The listing builds one solid part. Answer for the finished solid, in the listing's coordinates (mm). A direction names the side the tool comes from. Coordinates: 2 decimals unless noted, no trailing zeros. Loops run counter-clockwise (first coordinate to the right, second up) from the corner with the lowest first, then second, coordinate; pieces in that order, holes last. Notation, with made-up numbers: (26.5, 46.5) - (63.5, 46.5) arc R16 cw to (63.5, 69.5) - close; hole circle Ø7 at (-30, 51.25). An arc over 180 degrees is marked (long way). Put each result on its own line as item: value.
```python
from build123d import *

# Parameters (mm, degrees)
SKETCH1_W                = 25.4
SKETCH1_H                = 76.2
BOSS_EXTRUDE1_DEPTH      = 25.4
SKETCH2_W                = 22.225
SKETCH2_H                = 22.225
CUT_EXTRUDE1_DEPTH       = 138.235224905
BOSS_EXTRUDE2_DEPTH      = 3.175
BOSS_EXTRUDE2_DEPTH_BACK = 31.75
SKETCH3_R                = 12.7
SKETCH4_R                = 3.175
CUT_EXTRUDE3_DEPTH       = 104.653950262


with BuildPart() as part:
    # Sketch1 → Boss-Extrude1 (new body)
    with BuildSketch(Plane(origin=(0, 0, 0), x_dir=(0, 0, -1), z_dir=(1, 0, 0))):
        Rectangle(SKETCH1_W, SKETCH1_H)
        Polygon((-12.7, -44.45), (-12.7, -38.1), (-12.7, 38.1), (-12.7, 63.5), (-14.2875, 63.5), (-14.2875, -44.45), align=None)
        Polygon((-12.7, -44.45), (-22.225, -94.650277885), (-23.784673135, -94.354345527), (-14.2875, -44.45), align=None)
        Polygon((22.225, -94.650277885), (23.784673135, -94.354345527), (14.2875, -44.45), (12.7, -44.45), align=None)
        Polygon((12.7, -38.1), (12.7, -44.45), (14.2875, -44.45), (14.2875, 63.5), (12.7, 63.5), (12.7, 38.1), align=None)
    extrude(amount=BOSS_EXTRUDE1_DEPTH)

    # Sketch2 → Cut-Extrude1 (cut, through all)
    with BuildSketch(Plane(origin=(0, 38.1, 0), x_dir=(1, 0, 0), z_dir=(0, 1, 0))):
        with Locations((12.7, 0)):
            Rectangle(SKETCH2_W, SKETCH2_H)
    extrude(amount=-CUT_EXTRUDE1_DEPTH, mode=Mode.SUBTRACT)

    # Sketch3 → Boss-Extrude2 (add, two sides: drawn at the far end of the back side and taken through both)
    with BuildSketch(Plane(origin=(25.4, 0, 0), x_dir=(0, 0, -1), z_dir=(1, 0, 0)).offset(-BOSS_EXTRUDE2_DEPTH_BACK)):
        with Locations((0, -12.7)):
            Circle(SKETCH3_R)
    extrude(amount=BOSS_EXTRUDE2_DEPTH + BOSS_EXTRUDE2_DEPTH_BACK)

    # Sketch4 → Cut-Extrude3 (cut, through all)
    with BuildSketch(Plane(origin=(28.575, 0, 0), x_dir=(0, 0, -1), z_dir=(1, 0, 0))):
        with Locations((0, -12.7)):
            Circle(SKETCH4_R)
    extrude(amount=-CUT_EXTRUDE3_DEPTH, mode=Mode.SUBTRACT)


solid = part.part
```
1) For a pull along Z with two mould halves and no side action, classify faces 4 (the face through (12.522, -69.752, 19.103)), 5 (the face through (13, -41, -12.7)), 6 (the face through (28.575, -15, -3)), 7 (the face through (12.522, -69.752, -19.103)) as pulls with the +Z half, pulls with the -Z half, needs draft (parallel to the pull), parting line crosses it, or undercut.
Found:
face 4: pulls with the +Z half
face 5: undercut
face 6: needs draft
face 7: pulls with the -Z half
2) The part is cut by section C-C (y = 30). Give the vertices of the cut face in (x, z), and give its area (3 significant figures).
Found:
outline: (0, -14.29) - (25.4, -14.29) - (25.4, 14.29) - (0, 14.29) - close; hole (1.59, -11.11) - (23.81, -11.11) - (23.81, 11.11) - (1.59, 11.11) - close
area: 232 mm^2
3) Straight lines are drawn through the part: L1, parallel to Z at x = 8, y = 19; L2, parallel to X at y = 14, z = 5; L3, parallel to X at y = 31, z = 14. For each, find the intervals that lie inside material, in ascending order. Write a range as [from, to].
Found:
L1: z = [-14.29, -11.11], [11.11, 14.29]
L2: x = [0, 1.59], [23.81, 25.4]
L3: x = [0, 25.4]
4) Each of these flat-tipped pins is pushed along its axis until it touches: pin 1 (2 mm diameter, centred on x = 15.5, z = -1.5, fed in from +Y); pin 2 (9.5 mm diameter, centred on x = 17, y = -25, fed in from +Z); pin 3 (20.5 mm diameter, centred on x = 8, y = 54.5, fed in from -Z); pin 4 (14.5 mm diameter, centred on y = -25.5, z = -5.5, fed in from +X) (3 decimals). Where does it stop, or does it pass through?
Found:
pin 1: stops at y = -0.01
pin 2: stops at z = 14.29
pin 3: stops at z = -14.29
pin 4: stops at x = 28.575
5) For faces 1 (the face through (27, -20.4, 10.1)), 2 (the face through (13, 10, 14.288)), 3 (the face through (12.522, -69.199, -17.396)), determine the directions among +Z, -Z, +X, -X, +Y, -Y from which every point of the face is accessible in a straight line to the end or side of a thin tool.
Found:
face 1: +X
face 2: +Z, +X, -X, +Y
face 3: +X, -X, -Y
